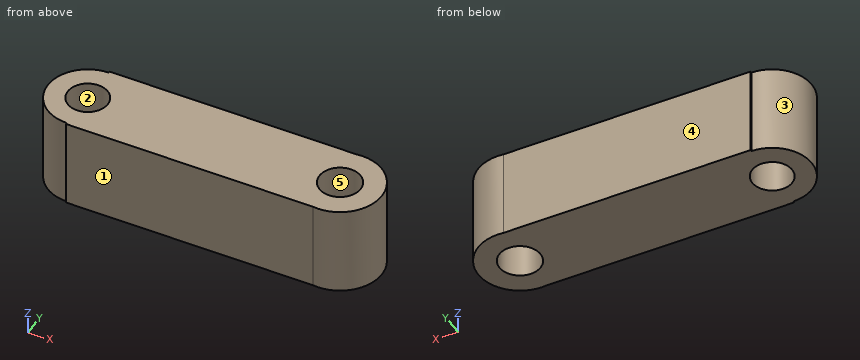
```python
from build123d import *

# Parameters (mm, degrees)
F0_R     = 8.6737376807
F1_DEPTH = 25.4
F0_R_2   = 8.4076501903
F2_DEPTH = 38.1


# Not quite as in the source:
# - a feature names something its author has since deleted; it is built from what else it names


with BuildPart() as f1:
    # F0 (on Top) → F1 (new body)
    with BuildSketch(Plane.XY):
        with BuildLine():
            ThreePointArc((51.0823471633, -17.43234694), (70.9533001066, 0), (51.0823471633, 17.43234694))
            Line((51.0823471633, 17.43234694), (-53.3713176847, 17.43234694))
            Line((-53.3713176847, 17.43234694), (-53.3713176847, 16.7665737877))
            ThreePointArc((-53.3713176847, 16.7665737877), (-41.5155596621, 11.8557580225), (-36.604743897, 0))
            ThreePointArc((-36.604743897, 0), (-41.5155596621, -11.8557580225), (-53.3713176847, -16.7665737877))
            Line((-53.3713176847, -16.7665737877), (-53.3713176847, -17.43234694))
            Line((-53.3713176847, -17.43234694), (51.0823471633, -17.43234694))
        make_face()
        with Locations((53.3713176847, 0)):
            Circle(F0_R, mode=Mode.SUBTRACT)
    extrude(amount=F1_DEPTH)

    # F0 (on Top) → F2 (join)
    with BuildSketch(Plane.XY):
        with BuildLine():
            ThreePointArc((51.0823471633, -17.43234694), (70.9533001066, 0), (51.0823471633, 17.43234694))
            Line((51.0823471633, 17.43234694), (-53.3713176847, 17.43234694))
            Line((-53.3713176847, 17.43234694), (-53.3713176847, 16.7665737877))
            ThreePointArc((-53.3713176847, 16.7665737877), (-41.5155596621, 11.8557580225), (-36.604743897, 0))
            ThreePointArc((-36.604743897, 0), (-41.5155596621, -11.8557580225), (-53.3713176847, -16.7665737877))
            Line((-53.3713176847, -16.7665737877), (-53.3713176847, -17.43234694))
            Line((-53.3713176847, -17.43234694), (51.0823471633, -17.43234694))
        make_face()
        with Locations((53.3713176847, 0)):
            Circle(F0_R, mode=Mode.SUBTRACT)
        with BuildLine():
            ThreePointArc((-36.604743897, 0), (-41.5155596621, 11.8557580225), (-53.3713176847, 16.7665737877))
            ThreePointArc((-53.3713176847, 16.7665737877), (-70.1378914723, 0), (-53.3713176847, -16.7665737877))
            ThreePointArc((-53.3713176847, -16.7665737877), (-41.5155596621, -11.8557580225), (-36.604743897, 0))
        make_face()
        with Locations((-53.3713176847, 0)):
            Circle(F0_R_2, mode=Mode.SUBTRACT)
    extrude(amount=F2_DEPTH)


solid = f1.part
```
Verification items for the finished model (mm, model axes). Face numbers are marked on the shaded views. A direction names the side the tool comes from. Coordinates: 2 decimals unless noted, no trailing zeros. Loops run counter-clockwise (first coordinate to the right, second up) from the corner with the lowest first, then second, coordinate; pieces in that order, holes last. Notation, with made-up numbers: (65.25, 55) -> (100.25, 55) arc R25 ccw to (100.25, 91) -> close; hole circle Ø6 at (-4.5, 27.5). An arc over 180 degrees is marked (long way). Answer in a Markdown table with one row per item. Add a question column.
1. Depth check by flat-ended pin: P1, Ø19, axis at x = -15.5, z = 11.5, coming from the -Y side; P2, Ø1, axis at y = -2, z = 20.5, coming from the -X side; P3, Ø1.5, axis at y = -2, z = 33, coming from the +X side; P4, Ø6, axis at x = 19, y = 6.5, coming from the -Z side. Enter the tip coordinate at first touch or a pass-through.
2. Access from +Z, -Z, +X, -X, +Y, -Y to the whole of each face (thin tool, end or side, straight path). Record for the marked faces 1 and 2.
3. Section check B-B, the plane z = 32.5. Enter the section's corners in (x, y), then the cut area to 3 significant figures.
4. Material ranges on probe 1 along X at (y, z) = (6.5, 12); probe 2 along X at (y, z) = (-6, 11) (3 decimals); probe 3 along Y at (x, z) = (-16.5, 23.5), recorded low to high. Write a range as [from, to].
5. Section check C-C, the plane x = -60.5. Enter the section's corners in (y, z), then the cut area to 3 significant figures.
6. Section check A-A, the plane y = 0. Enter the section's corners in (x, z), then the cut area to 3 significant figures.
7. Draft check along X on the marked faces 3, 4 and 5. Enter one of: +X half, -X half, draft (parallel to the pull), parting line (faces both ways), or undercut.
Derived:
| question | item | result |
|---|---|---|
| 1 | P1 | stops at y = -17.43 |
| 1 | P2 | stops at x = -70.07 |
| 1 | P3 | stops at x = 70.91 |
| 1 | P4 | stops at z = 0 |
| 2 | face 1 | +Z, -Z, -X, -Y |
| 2 | face 2 | +Z, -Z |
| 3 | outline | (-53.37, -17.43) -> (51.08, -17.43) arc R17.58 ccw (long way) to (51.08, 17.43) -> (-53.37, 17.43) -> (-53.37, 16.77) arc R16.77 ccw to (-53.37, -16.77) -> close; hole circle Ø16.82 at (-53.37, 0); hole circle Ø17.35 at (53.37, 0) |
| 3 | area | 4,190 mm² |
| 4 | probe 1 | x = [-68.83, -58.7], [-48.04, 47.63], [59.11, 69.71] |
| 4 | probe 2 | x = [-69.028, -59.261], [-47.482, 47.108], [59.635, 69.898] |
| 4 | probe 3 | y = [-17.43, 17.43] |
| 5 | outline | (-15.18, 0) -> (-4.46, 0) -> (-4.46, 38.1) -> (-15.18, 38.1) -> close; (4.46, 0) -> (15.18, 0) -> (15.18, 38.1) -> (4.46, 38.1) -> close |
| 5 | area | 817 mm² |
| 6 | outline | (-70.14, 0) -> (-61.78, 0) -> (-61.78, 38.1) -> (-70.14, 38.1) -> close; (-44.96, 0) -> (44.7, 0) -> (44.7, 38.1) -> (-44.96, 38.1) -> close; (62.05, 0) -> (70.95, 0) -> (70.95, 38.1) -> (62.05, 38.1) -> close |
| 6 | area | 4,070 mm² |
| 7 | face 3 | -X half |
| 7 | face 4 | draft |
| 7 | face 5 | undercut |
